For this review, take the finished solid that the model builds, in its own axes (mm). Give positions to 0.01 mm unless a question says otherwise; leave off trailing zeros. Return JSON: item names as keys, results as strings. Group by question number.
1) To check wall thickness, follow line 1 along Y through (x, z) = (0, 45.5); line 2 along Y through (x, z) = (-1.75, 54.5); line 3 along Y through (x, z) = (-6.75, -33). State the ranges of each line that lie inside material, in increasing order.
2) The part is to be moulded in two halves that separate along Y. For faces 1 (the face through (2.483, 0.782, 2.045)), 2 (the face through (0, 3, 146.05)), say which applies: released by +Y, released by -Y, zero draft, split by the parting line, or undercut.
3) Insertion check: P1, Ø4, axis at y = 1, z = -10.5, coming from the +X side; P2, Ø7, axis at x = 0, y = 0, coming from the +Z side; P3, Ø1.5, axis at y = 3.5, z = 94.5, coming from the -X side; P4, Ø1.9, axis at x = -1, z = -49.5, coming from the +Y side. Each pin has a flat end and moves straight along its axis. Give the tip position at first contact, or say it passes through.
from build123d import *

# Parameters (mm, degrees)
SKETCH3_W                = 25.4
SKETCH3_H                = 25.4
BOSS_EXTRUDE1_DEPTH      = 146.05
BOSS_EXTRUDE1_DEPTH_BACK = 146.05
SKETCH4_R                = 2.6035
CUT_EXTRUDE1_DEPTH       = 293.1
CUT_EXTRUDE2_DEPTH       = 293.1
FILLET1_R                = 2.54
FILLET2_R                = 1.778


with BuildPart() as part:
    # Sketch3 → Boss-Extrude1 (new body, two sides)
    with BuildSketch(Plane.XY) as boss_extrude1_sk:
        Rectangle(SKETCH3_W, SKETCH3_H)
    extrude(amount=BOSS_EXTRUDE1_DEPTH)
    extrude(boss_extrude1_sk.sketch, amount=-BOSS_EXTRUDE1_DEPTH_BACK)

    # Sketch4 → Cut-Extrude1 (cut, through all)
    with BuildSketch(Plane.XY.offset(146.05)):
        with BuildLine():
            Line((3.2512, 12.7), (-3.2512, 12.7))
            Line((-3.2512, 12.7), (-3.2512, 10.4902))
            Line((-3.2512, 10.4902), (-6.348478019, 10.4902))
            ThreePointArc((-6.348478019, 10.4902), (-7.335478831, 9.830707141), (-7.103895736, 8.666460301))
            Line((-7.103895736, 8.666460301), (-2.958635435, 4.5212))
            Line((-2.958635435, 4.5212), (2.958635435, 4.5212))
            Line((2.958635435, 4.5212), (7.103895736, 8.666460301))
            ThreePointArc((7.103895736, 8.666460301), (7.335478831, 9.830707141), (6.348478019, 10.4902))
            Line((6.348478019, 10.4902), (3.2512, 10.4902))
            Line((3.2512, 10.4902), (3.2512, 12.7))
        make_face()
        with BuildLine():
            Line((12.7, -3.2512), (12.7, 3.2512))
            Line((12.7, 3.2512), (10.4902, 3.2512))
            Line((10.4902, 3.2512), (10.4902, 6.348478019))
            ThreePointArc((10.4902, 6.348478019), (9.830707141, 7.335478831), (8.666460301, 7.103895736))
            Line((8.666460301, 7.103895736), (4.5212, 2.958635435))
            Line((4.5212, 2.958635435), (4.5212, -2.958635435))
            Line((4.5212, -2.958635435), (8.666460301, -7.103895736))
            ThreePointArc((8.666460301, -7.103895736), (9.830707141, -7.335478831), (10.4902, -6.348478019))
            Line((10.4902, -6.348478019), (10.4902, -3.2512))
            Line((10.4902, -3.2512), (12.7, -3.2512))
        make_face()
        with BuildLine():
            Line((-3.2512, -10.4902), (-3.2512, -12.7))
            Line((-3.2512, -12.7), (3.2512, -12.7))
            Line((3.2512, -12.7), (3.2512, -10.4902))
            Line((3.2512, -10.4902), (6.348478019, -10.4902))
            ThreePointArc((6.348478019, -10.4902), (7.335478831, -9.830707141), (7.103895736, -8.666460301))
            Line((7.103895736, -8.666460301), (2.958635435, -4.5212))
            Line((2.958635435, -4.5212), (-2.958635435, -4.5212))
            Line((-2.958635435, -4.5212), (-7.103895736, -8.666460301))
            ThreePointArc((-7.103895736, -8.666460301), (-7.335478831, -9.830707141), (-6.348478019, -10.4902))
            Line((-6.348478019, -10.4902), (-3.2512, -10.4902))
        make_face()
        with BuildLine():
            Line((-10.4902, 3.2512), (-12.7, 3.2512))
            Line((-12.7, 3.2512), (-12.7, -3.2512))
            Line((-12.7, -3.2512), (-10.4902, -3.2512))
            Line((-10.4902, -3.2512), (-10.4902, -6.348478019))
            ThreePointArc((-10.4902, -6.348478019), (-9.830707141, -7.335478831), (-8.666460301, -7.103895736))
            Line((-8.666460301, -7.103895736), (-4.5212, -2.958635435))
            Line((-4.5212, -2.958635435), (-4.5212, 2.958635435))
            Line((-4.5212, 2.958635435), (-8.666460301, 7.103895736))
            ThreePointArc((-8.666460301, 7.103895736), (-9.830707141, 7.335478831), (-10.4902, 6.348478019))
            Line((-10.4902, 6.348478019), (-10.4902, 3.2512))
        make_face()
        Circle(SKETCH4_R)
    extrude(amount=-CUT_EXTRUDE1_DEPTH, mode=Mode.SUBTRACT)

    # Sketch5 → Cut-Extrude2 (cut, through all)
    with BuildSketch(Plane.XY.offset(146.05)):
        with BuildLine():
            ThreePointArc((-11.5951, 3.2512), (-12.376382283, 3.574817717), (-12.7, 4.3561))
            Line((-12.7, 4.3561), (-12.7, 3.2512))
            Line((-12.7, 3.2512), (-11.5951, 3.2512))
        make_face()
        with BuildLine():
            ThreePointArc((-10.4902, 4.3561), (-10.813817717, 3.574817717), (-11.5951, 3.2512))
            Line((-11.5951, 3.2512), (-10.4902, 3.2512))
            Line((-10.4902, 3.2512), (-10.4902, 4.3561))
        make_face()
        with BuildLine():
            Line((-12.7, -3.2512), (-12.7, -4.3561))
            ThreePointArc((-12.7, -4.3561), (-12.376382283, -3.574817717), (-11.5951, -3.2512))
            Line((-11.5951, -3.2512), (-12.7, -3.2512))
        make_face()
        with BuildLine():
            Line((-10.4902, -3.2512), (-11.5951, -3.2512))
            ThreePointArc((-11.5951, -3.2512), (-10.813817717, -3.574817717), (-10.4902, -4.3561))
            Line((-10.4902, -4.3561), (-10.4902, -3.2512))
        make_face()
        with BuildLine():
            Line((-3.2512, -11.595100007), (-3.2512, -10.4902))
            Line((-3.2512, -10.4902), (-4.3561, -10.4902))
            ThreePointArc((-4.3561, -10.4902), (-3.574817715, -10.81381772), (-3.2512, -11.595100007))
        make_face()
        with BuildLine():
            Line((-3.2512, -12.7), (-3.2512, -11.595100007))
            ThreePointArc((-3.2512, -11.595100007), (-3.57481772, -12.376382285), (-4.3561, -12.7))
            Line((-4.3561, -12.7), (-3.2512, -12.7))
        make_face()
        with BuildLine():
            Line((3.2512, -10.4902), (3.2512, -11.5951))
            ThreePointArc((3.2512, -11.5951), (3.574817718, -10.813817717), (4.3561, -10.4902))
            Line((4.3561, -10.4902), (3.2512, -10.4902))
        make_face()
        with BuildLine():
            Line((3.2512, -12.7), (4.3561, -12.7))
            ThreePointArc((4.3561, -12.7), (3.574817717, -12.376382282), (3.2512, -11.5951))
            Line((3.2512, -11.5951), (3.2512, -12.7))
        make_face()
        with BuildLine():
            Line((11.5951, -3.2512), (10.4902, -3.2512))
            Line((10.4902, -3.2512), (10.4902, -4.3561))
            ThreePointArc((10.4902, -4.3561), (10.813817717, -3.574817717), (11.5951, -3.2512))
        make_face()
        with BuildLine():
            Line((12.7, -3.2512), (11.5951, -3.2512))
            ThreePointArc((11.5951, -3.2512), (12.376382283, -3.574817717), (12.7, -4.3561))
            Line((12.7, -4.3561), (12.7, -3.2512))
        make_face()
        with BuildLine():
            Line((10.4902, 3.2512), (11.5951, 3.2512))
            ThreePointArc((11.5951, 3.2512), (10.813817717, 3.574817717), (10.4902, 4.3561))
            Line((10.4902, 4.3561), (10.4902, 3.2512))
        make_face()
        with BuildLine():
            Line((12.7, 3.2512), (12.7, 4.3561))
            ThreePointArc((12.7, 4.3561), (12.376382283, 3.574817717), (11.5951, 3.2512))
            Line((11.5951, 3.2512), (12.7, 3.2512))
        make_face()
        with BuildLine():
            Line((3.2512, 12.7), (3.2512, 11.595099996))
            ThreePointArc((3.2512, 11.595099996), (3.574817716, 12.376382281), (4.3561, 12.7))
            Line((4.3561, 12.7), (3.2512, 12.7))
        make_face()
        with BuildLine():
            Line((3.2512, 11.595099996), (3.2512, 10.4902))
            Line((3.2512, 10.4902), (4.3561, 10.4902))
            ThreePointArc((4.3561, 10.4902), (3.574817719, 10.813817716), (3.2512, 11.595099996))
        make_face()
        with BuildLine():
            Line((-3.2512, 12.7), (-4.3561, 12.7))
            ThreePointArc((-4.3561, 12.7), (-3.574817717, 12.376382283), (-3.2512, 11.5951))
            Line((-3.2512, 11.5951), (-3.2512, 12.7))
        make_face()
        with BuildLine():
            Line((-3.2512, 10.4902), (-3.2512, 11.5951))
            ThreePointArc((-3.2512, 11.5951), (-3.574817717, 10.813817717), (-4.3561, 10.4902))
            Line((-4.3561, 10.4902), (-3.2512, 10.4902))
        make_face()
        with BuildLine():
            ThreePointArc((-12.7, 5.23875), (-12.14755, 5.7912), (-12.7, 6.34365))
            Line((-12.7, 6.34365), (-12.7, 5.23875))
        make_face()
        with BuildLine():
            ThreePointArc((-12.7, 9.60755), (-12.14755, 10.16), (-12.7, 10.71245))
            Line((-12.7, 10.71245), (-12.7, 9.60755))
        make_face()
        with BuildLine():
            ThreePointArc((-10.71245, 12.7), (-10.16, 12.14755), (-9.60755, 12.7))
            Line((-9.60755, 12.7), (-10.71245, 12.7))
        make_face()
        with BuildLine():
            ThreePointArc((-6.34365, 12.7), (-5.7912, 12.14755), (-5.23875, 12.7))
            Line((-5.23875, 12.7), (-6.34365, 12.7))
        make_face()
        with BuildLine():
            Line((6.34365, 12.7), (5.23875, 12.7))
            ThreePointArc((5.23875, 12.7), (5.7912, 12.14755), (6.34365, 12.7))
        make_face()
        with BuildLine():
            Line((10.71245, 12.7), (9.60755, 12.7))
            ThreePointArc((9.60755, 12.7), (10.16, 12.14755), (10.71245, 12.7))
        make_face()
        with BuildLine():
            Line((12.7, 10.71245), (12.7, 9.60755))
            ThreePointArc((12.7, 9.60755), (12.14755, 10.16), (12.7, 10.71245))
        make_face()
        with BuildLine():
            Line((12.7, 6.34365), (12.7, 5.23875))
            ThreePointArc((12.7, 5.23875), (12.14755, 5.7912), (12.7, 6.34365))
        make_face()
        with BuildLine():
            Line((-12.7, -6.34365), (-12.7, -5.23875))
            ThreePointArc((-12.7, -5.23875), (-12.14755, -5.7912), (-12.7, -6.34365))
        make_face()
        with BuildLine():
            Line((-12.7, -10.71245), (-12.7, -9.60755))
            ThreePointArc((-12.7, -9.60755), (-12.14755, -10.16), (-12.7, -10.71245))
        make_face()
        with BuildLine():
            Line((-10.71245, -12.7), (-9.60755, -12.7))
            ThreePointArc((-9.60755, -12.7), (-10.16, -12.14755), (-10.71245, -12.7))
        make_face()
        with BuildLine():
            Line((-6.34365, -12.7), (-5.23875, -12.7))
            ThreePointArc((-5.23875, -12.7), (-5.7912, -12.14755), (-6.34365, -12.7))
        make_face()
        with BuildLine():
            Line((12.7, -10.71245), (12.7, -9.60755))
            ThreePointArc((12.7, -9.60755), (12.14755, -10.16), (12.7, -10.71245))
        make_face()
        with BuildLine():
            Line((12.7, -6.34365), (12.7, -5.23875))
            ThreePointArc((12.7, -5.23875), (12.14755, -5.7912), (12.7, -6.34365))
        make_face()
        with BuildLine():
            Line((10.71245, -12.7), (9.60755, -12.7))
            ThreePointArc((9.60755, -12.7), (10.16, -12.14755), (10.71245, -12.7))
        make_face()
        with BuildLine():
            Line((6.34365, -12.7), (5.23875, -12.7))
            ThreePointArc((5.23875, -12.7), (5.7912, -12.14755), (6.34365, -12.7))
        make_face()
    extrude(amount=-CUT_EXTRUDE2_DEPTH, mode=Mode.SUBTRACT)

    # Fillet1
    fillet1_edges = [part.edges().sort_by_distance(p)[0] for p in [
        (2.958635435, 4.5212, 0),
        (-2.958635435, 4.5212, 0),
        (-2.958635435, -4.5212, 0),
        (2.958635435, -4.5212, 0),
        (4.5212, -2.958635435, 0),
        (4.5212, 2.958635435, 0),
        (-4.5212, 2.958635435, 0),
        (-4.5212, -2.958635435, 0),
    ]]
    fillet(fillet1_edges, radius=FILLET1_R)

    # Fillet2
    fillet2_edges = [part.edges().sort_by_distance(p)[0] for p in [
        (-12.7, 12.7, 0),
        (12.7, 12.7, 0),
        (12.7, -12.7, 0),
        (-12.7, -12.7, 0),
    ]]
    fillet(fillet2_edges, radius=FILLET2_R)


solid = part.part
Evaluation:
{
 "1": {"line 1": "-4.52 to -2.6, 2.6 to 4.52", "line 2": "-4.52 to -1.93, 1.93 to 4.52", "line 3": "-12.7 to -10.41, -8.31 to -5.19, 5.19 to 8.31, 10.41 to 12.7"},
 "2": {"face 1": "undercut", "face 2": "zero draft"},
 "3": {"P1": "x = 4.77", "P2": "z = 146.05", "P3": "x = -12.69", "P4": "y = 4.52"}
}
